Model file for the job. Use its own axes, mm. A direction names the side the tool comes from. Round coordinates to 2 decimals unless told otherwise and drop trailing zeros. Loops run counter-clockwise (first coordinate to the right, second up) from the corner with the lowest first, then second, coordinate; pieces in that order, holes last. Notation, with made-up numbers: (75.5, -18) -> (92.5, -18) arc R16 ccw to (92.5, -13) -> close; hole circle Ø4 at (44.5, 6.5). An arc over 180 degrees is marked (long way). Use a Markdown table: item, result.
from build123d import *

# Parameters (mm, degrees)
F1_DEPTH = 20
F3_D     = 5.5
F5_D     = 5.5
F7_DEPTH = 30


# Not quite as in the source:
# - after a boolean that leaves OpenCascade's solid faulty, fix() repairs it


with BuildPart() as f1:
    # F0 (on Top) → F1 (new body)
    with BuildSketch(Plane.XY):
        with BuildLine():
            Line((37.1651718683, -5), (37.1651718683, 5))
            ThreePointArc((37.1651718683, 5), (26.5165042945, 26.5165042945), (5, 37.1651718683))
            Line((5, 37.1651718683), (-5, 37.1651718683))
            ThreePointArc((-5, 37.1651718683), (-26.5165042945, 26.5165042945), (-37.1651718683, 5))
            Line((-37.1651718683, 5), (-37.1651718683, -5))
            ThreePointArc((-37.1651718683, -5), (-26.5165042945, -26.5165042945), (-5, -37.1651718683))
            Line((-5, -37.1651718683), (5, -37.1651718683))
            ThreePointArc((5, -37.1651718683), (26.5165042945, -26.5165042945), (37.1651718683, -5))
        make_face()
        with BuildLine():
            ThreePointArc((-5, -34.1357583774), (-24.3951839509, -24.3951839509), (-34.1357583774, -5))
            Line((-34.1357583774, -5), (-34.1357583774, 5))
            ThreePointArc((-34.1357583774, 5), (-24.3951839509, 24.3951839509), (-5, 34.1357583774))
            Line((-5, 34.1357583774), (5, 34.1357583774))
            ThreePointArc((5, 34.1357583774), (24.3951839509, 24.3951839509), (34.1357583774, 5))
            Line((34.1357583774, 5), (34.1357583774, -5))
            ThreePointArc((34.1357583774, -5), (24.3951839509, -24.3951839509), (5, -34.1357583774))
            Line((5, -34.1357583774), (-5, -34.1357583774))
        make_face(mode=Mode.SUBTRACT)
    extrude(amount=F1_DEPTH)

    # F3 (through all)
    with Locations(Plane.YZ.offset(37.1651718683)):
        with Locations((0, 10)):
            Hole(F3_D / 2)

    # F5 (through all)
    with Locations(Plane.XZ.offset(37.1651718683)):
        with Locations((0, 10)):
            Hole(F5_D / 2)

    # F6 (on face) → F7 (join)
    with BuildSketch(Plane(origin=(0, 0, 0), x_dir=(1, 0, 0), z_dir=(0, 0, -1))):
        with BuildLine():
            Line((37.1651718683, -5), (37.1651718683, 5))
            ThreePointArc((37.1651718683, 5), (26.5165042945, 26.5165042945), (5, 37.1651718683))
            Line((5, 37.1651718683), (-5, 37.1651718683))
            ThreePointArc((-5, 37.1651718683), (-26.5165042945, 26.5165042945), (-37.1651718683, 5))
            Line((-37.1651718683, 5), (-37.1651718683, -5))
            ThreePointArc((-37.1651718683, -5), (-26.5165042945, -26.5165042945), (-5, -37.1651718683))
            Line((-5, -37.1651718683), (5, -37.1651718683))
            ThreePointArc((5, -37.1651718683), (26.5165042945, -26.5165042945), (37.1651718683, -5))
        make_face()
        with BuildLine():
            ThreePointArc((34.1357583774, 5), (34.4088191022, 2.5066248203), (34.5, 0))
            ThreePointArc((34.5, 0), (34.4088191022, -2.5066248203), (34.1357583774, -5))
            ThreePointArc((34.1357583774, -5), (24.3951839509, -24.3951839509), (5, -34.1357583774))
            ThreePointArc((5, -34.1357583774), (0, -34.5), (-5, -34.1357583774))
            ThreePointArc((-5, -34.1357583774), (-24.3951839509, -24.3951839509), (-34.1357583774, -5))
            ThreePointArc((-34.1357583774, -5), (-34.5, 0), (-34.1357583774, 5))
            ThreePointArc((-34.1357583774, 5), (-24.3951839509, 24.3951839509), (-5, 34.1357583774))
            ThreePointArc((-5, 34.1357583774), (0, 34.5), (5, 34.1357583774))
            ThreePointArc((5, 34.1357583774), (24.3951839509, 24.3951839509), (34.1357583774, 5))
        make_face(mode=Mode.SUBTRACT)
        with BuildLine():
            Line((-5, 37.1651718683), (5, 37.1651718683))
            ThreePointArc((5, 37.1651718683), (0, 37.5), (-5, 37.1651718683))
        make_face()
        with BuildLine():
            ThreePointArc((37.1651718683, -5), (37.4161993331, -2.5055992236), (37.5, 0))
            ThreePointArc((37.5, 0), (37.4161993331, 2.5055992236), (37.1651718683, 5))
            Line((37.1651718683, 5), (37.1651718683, -5))
        make_face()
        with BuildLine():
            ThreePointArc((-5, -37.1651718683), (0, -37.5), (5, -37.1651718683))
            Line((5, -37.1651718683), (-5, -37.1651718683))
        make_face()
        with BuildLine():
            Line((-37.1651718683, -5), (-37.1651718683, 5))
            ThreePointArc((-37.1651718683, 5), (-37.5, 0), (-37.1651718683, -5))
        make_face()
    extrude(amount=F7_DEPTH)

    add(f1.part.fix(), mode=Mode.REPLACE)


solid = f1.part
Q1. Band-saw the part on B-B, the plane x = 0. Give the cut face in (y, z).
Results list:
| item | result |
|---|---|
| outline | (-37.5, -30) -> (-34.5, -30) -> (-34.5, 0) -> (-34.14, 0) -> (-34.14, 7.25) -> (-37.17, 7.25) -> (-37.17, 0) -> (-37.5, 0) -> close; (-37.17, 12.75) -> (-34.14, 12.75) -> (-34.14, 20) -> (-37.17, 20) -> close; (34.14, 0) -> (34.5, 0) -> (34.5, -30) -> (37.5, -30) -> (37.5, 0) -> (37.17, 0) -> (37.17, 7.25) -> (34.14, 7.25) -> close; (34.14, 12.75) -> (37.17, 12.75) -> (37.17, 20) -> (34.14, 20) -> close |
Q2. Band-saw the part on C-C, the plane y = 7.5. Give the cut face in (x, z), plus the area to 3 significant figures.
Results list:
| item | result |
|---|---|
| outline | (-36.74, -30) -> (-33.67, -30) -> (-33.67, 20) -> (-36.74, 20) -> close; (33.67, -30) -> (36.74, -30) -> (36.74, 20) -> (33.67, 20) -> close |
| area | 307 mm² |
Q3. Band-saw the part on D-D, the plane x = -17.5. Give the cut face in (y, z), plus the area to 3 significant figures.
Results list:
| item | result |
|---|---|
| outline | (-33.17, -30) -> (-29.73, -30) -> (-29.73, 20) -> (-33.17, 20) -> close; (29.73, -30) -> (33.17, -30) -> (33.17, 20) -> (29.73, 20) -> close |
| area | 343 mm² |
Q4. Flat gauge pins, fed straight in: pin 1 (3 mm diameter, centred on y = -1, z = 12, fed in from +X); pin 2 (8 mm diameter, centred on x = -16, y = 24.5, fed in from -Z); pin 3 (6.5 mm diameter, centred on x = 0, z = 10, fed in from +Y); pin 4 (4 mm diameter, centred on x = 8.5, z = -18.5, fed in from +Y). Where does each tip first touch, or does it go through?
Results list:
| item | result |
|---|---|
| pin 1 | stops at x = 37.17 |
| pin 2 | passes through |
| pin 3 | stops at y = 37.17 |
| pin 4 | stops at y = 36.93 |
Q5. Tool access for faces 1 (the face through (2.2, 34.136, 7.6)), 2 (the face through (-37.165, -2.2, 7.6)), 3 (the face through (11, 33, -30)): list every direction of +Z, -Z, +X, -X, +Y, -Y with a clear straight run to the whole face (end or side of a thin tool).
Results list:
| item | result |
|---|---|
| face 1 | +Z, -Z |
| face 2 | +Z, -X, +Y, -Y |
| face 3 | -Z, +X, -X, +Y, -Y |
Q6. Drill centre lines: L1, parallel to Z at x = 0, y = -36.25; L2, parallel to X at y = -5, z = 14. Where is each one in solid material? Low to high. Write a range as from..to.
Results list:
| item | result |
|---|---|
| L1 | z = -30..7.25, 12.75..20 |
| L2 | x = -37.17..-34.14, 34.14..37.17 |
Q7. Band-saw the part on A-A, the plane z = 1. Give the cut face in (x, y), plus the area to 3 significant figures.
Results list:
| item | result |
|---|---|
| outline | (-37.17, -5) arc R37.5 ccw to (-5, -37.17) -> (5, -37.17) arc R37.5 ccw to (37.17, -5) -> (37.17, 5) arc R37.5 ccw to (5, 37.17) -> (-5, 37.17) arc R37.5 ccw to (-37.17, 5) -> close; hole (-34.14, -5) arc R34.5 ccw to (-5, -34.14) -> (5, -34.14) arc R34.5 ccw to (34.14, -5) -> (34.14, 5) arc R34.5 ccw to (5, 34.14) -> (-5, 34.14) arc R34.5 ccw to (-34.14, 5) -> close |
| area | 679 mm² |
Q8. Pull direction Y, two halves, no side cores. Call faces 4 (the face through (2.2, -37.165, 7.6)), 5 (the face through (37.165, 2.2, 7.6)), 6 (the face through (-2.2, 37.165, 7.6)), 7 (the face through (35.629, 0.358, 12.727)): released by +Y, released by -Y, zero draft, split by the parting line, or undercut.
Results list:
| item | result |
|---|---|
| face 4 | released by -Y |
| face 5 | zero draft |
| face 6 | released by +Y |
| face 7 | undercut |
